Source: CAD feature listing. Evaluate the final solid. Frame: model axes, mm. A direction names the side the tool comes from. Coordinates: 2 decimals unless noted, no trailing zeros. Order: outer loops, then holes, each group sorted by start corner. A loop starts at its lowest first (then second) coordinate and runs counter-clockwise, first axis right, second up.
Item 1: Ray query, line 1 (X direction, y = 3.75, z = -4.25); line 2 (Z direction, x = 52, y = 0). Return the intervals inside material, ascending.
Item 2: Contact query for flat-ended pins moving along their axis: P1, Ø8, axis at x = 6.5, y = -3, coming from the +Z side; P2, Ø1.5, axis at x = 1.5, y = 3.5, coming from the -Z side; P3, Ø6, axis at y = 6.5, z = 5, coming from the +X side; P4, Ø6.5, axis at y = -5, z = 0.5, coming from the +X side. Output: stop coordinate, or through.
Item 3: Reachability of faces 1 (the flat face through (-0.635, -7.5, -0.6)), 2 (the flat face through (-6.172, 0, 0)), 3 (the conical face through (-6.063, -7.325, 0.161)), 4 (the cylindrical face through (-0.31, -7.13, 0.31)), 5 (the flat face through (-0.635, 7.5, -0.6)) from +Z, -Z, +X, -X, +Y, -Y: full face, straight path, thin tool, end or side. Return the list, or none.
Item 4: Section A-A on x = -2. Return the cut outline in (y, z).
Item 5: Section B-B on x = 53.5. Return the cut outline in (y, z) (1 decimal).
Autodesk Inventor part; units mm, degrees
ref_plane "Work Plane1" through (1.525, 0, 0) normal (0, 0, 1) x (1, 0, 0)
ref_plane "YZ Plane" through (0, 0, 0) normal (1, 0, 0) x (0, 1, 0)
ref_plane "XZ Plane" through (0, 0, 0) normal (0, 1, 0) x (-1, 0, 0)
sketch "Sketch1" plane through (0, 0, 0) normal (0, 0, 1) x (1, 0, 0)
  line L0 (0, 7.1374) -> (0, 4.7625)
  line L1 (31.75, 4.7625) -> (57.15, 4.7625)
  line L2 (57.15, 4.7625) -> (57.15, 0)
  line L3 (57.15, 0) -> (-0.6351, 0)
  line L4 (-12.1921, 0) -> (68.707, 0)
  line L5 (-0.6351, 0) -> (-0.6351, 7.1374)
  line L6 (-0.6351, 7.1374) -> (0, 7.1374)
  line L7 (31.75, 4.7625) -> (20.6247, 4.7625)
  line L8 (20.6247, 4.7625) -> (0, 4.7625)
  line L9 (0, -1.4275) -> (0, 8.5649)
  dimension "d0" = 57.15
  dimension "d1" = 25.4
  dimension "d2" = 9.525
  dimension "d9" = 0.6351
  dimension "d10" = 14.2748
  dimension "d13" = 11.1253
  dimension "d14" = 9.525
revolve "Body" add sketch "Sketch1" angle 360 about axis through (57.15, 0, 0) along (-1, 0, 0)
sketch "Sketch2" plane through (-0.6351, 0, 0) normal (-1, 0, 0) x (0, 0, 1)
  line L0 (0, 8.2416) -> (7.1374, 4.1208)
  line L1 (7.1374, 4.1208) -> (7.1374, -4.1208)
  line L2 (7.1374, -4.1208) -> (0, -8.2416)
  line L3 (0, -8.2416) -> (-7.1374, -4.1208)
  line L4 (-7.1374, -4.1208) -> (-7.1374, 4.1208)
  line L5 (-7.1374, 4.1208) -> (0, 8.2416)
  point P0 (0, 0)
  point P1 (0, 0)
  dimension "d11" = 14.2748
extrude "Head" add sketch "Sketch2" along normal blind 5.5372
sketch "Sketch4" plane through (0, 0, 0) normal (0, 0, 1) x (1, 0, 0)
  line L0 (-6.1723, 7.1374) -> (-6.1723, 8.2416)
  line L1 (-6.1723, 8.2416) -> (-5.5348, 8.2416)
  line L2 (-5.5348, 8.2416) -> (-6.1723, 7.1374)
  line L3 (-7.2797, 0) -> (0.4723, 0)
  line L4 (-0.6351, 8.2416) -> (-6.1723, 8.2416)
  line L5 (-6.1723, 4.1208) -> (-6.1723, 8.2416)
  dimension "d5" = 30
  dimension "d19" = 14.2748
revolve "Chamfer1" cut sketch "Sketch4" angle 360 about axis through (-10, 0, 0) along (1, 0, 0)
thread "Thread"
chamfer "Chamfer2" distance 0.9738 distance2 0.9739 1 edges at (57.15, -4.7625, 0) measured on face at (57.15, 0.9018, -1.6622)
ref_plane "Work Plane1" through (1.525, 0, 0) normal (0, 0, 1) x (1, 0, 0)
equation "\"d0\" = NLG"
equation "\"d1\" = GEL"
equation "\"d2\" = GD"
equation "\"d10\" = SD2"
equation "\"d14\" = BDM"
equation "\"d11\" = SW"
equation "\"d3\" = KOH - SD"
equation "\"d5\" = ANG1"
equation "\"d19\" = SW0"
equation "\"d15\" = GEL"
equation "\"d6\" = -0.5 * SPD + 0.5 * GD"
equation "\"NLG\" = 57.15"
equation "\"GD\" = 9.525"
equation "\"BDM\" = 9.525"
equation "\"KOH\" = 6.1722"
equation "\"GEL\" = 25.4"
equation "\"SW\" = 14.2748"
equation "\"SW0\" = SW"
equation "\"SPD\" = GD1"
equation "\"SD2\" = SW"
equation "\"SD\" = 0.635"
equation "\"ANG1\" = 30deg"
equation "\"GAL\" = 11.1252"
equation "\"GUL\" = 0.97384"
equation "\"RR\" = 0.381"
equation "\"WFT\" = SD"
equation "\"GD1\" = 7.57733"
equation "\"THREADDIA\" = 9.525"
equation "\"SDH\" = SW"
equation "\"SDHG\" = 20.6248"
equation "\"TOA\" = 30deg"
equation "\"FAWI\" = 45deg"
equation "\"NND\" = 9.525"
equation "\"E0\" = 16.48739"
properties part number "AS 2465 - 3/8 x 2 1/4  UNC" material "Steel, Mild"
Answer list:
1. line 1: x = -6.17 to 0
1. line 2: z = -4.76 to 4.76
2. P1: stops at z = 4.76
2. P2: stops at z = -3.89
2. P3: stops at x = 0
2. P4: stops at x = 57.15
3. face 1: +X, -Y
3. face 2: +Z, -Z, -X, +Y, -Y
3. face 3: -X, -Y
3. face 4: +X
3. face 5: +X, +Y
4. outline: (-8.24, 0) - (-4.12, -7.14) - (4.12, -7.14) - (8.24, 0) - (4.12, 7.14) - (-4.12, 7.14) - close
5. outline: circle Ø9.5 at (0, 0)
